from build123d import *

# Parameters (mm, degrees)
SKETCH001_W   = 60
SKETCH001_H   = 80
SKETCH001_W_2 = 56
SKETCH001_H_2 = 76
PAD_DEPTH     = 30


with BuildPart() as part:
    # Sketch001 → Pad (new body)
    with BuildSketch(Plane.XY.offset(2)):
        Rectangle(SKETCH001_W, SKETCH001_H)
        Rectangle(SKETCH001_W_2, SKETCH001_H_2, mode=Mode.SUBTRACT)
    extrude(amount=PAD_DEPTH)


solid = part.part
The listing builds one solid part. Answer for the finished solid, in the listing's coordinates (mm). A direction names the side the tool comes from. Coordinates: 2 decimals unless noted, no trailing zeros. Loops run counter-clockwise (first coordinate to the right, second up) from the corner with the lowest first, then second, coordinate; pieces in that order, holes last. Notation, with made-up numbers: (50.25, -39) -> (100.25, -39) arc R14 ccw to (100.25, -13) -> close; hole circle Ø3 at (12.5, 72). An arc over 180 degrees is marked (long way). Write item = value, one per line. Start each with the question number.
1) Straight lines are drawn through the part: line 1 (Y direction, x = -4, z = 15.5); line 2 (X direction, y = 20.5, z = 12.75). For each, find the intervals that lie inside material, in ascending order. Write a range as from..to.
2) A cutting plane is placed at A-A (z = 23.5). Give the vertices of the cut face in (x, y).
3) A tool of negligible diameter and unlimited length cuts with its end or side. For faces 1 (the face through (28, -1, 17)), 2 (the face through (-29, 0, 2)), from which of +Z, -Z, +X, -X, +Y, -Y can it reach the whole face along a straight path? Write none if from no direction.
4) A cutting plane is placed at B-B (x = -14.5). Give the vertices of the cut face in (y, z).
5) The mould has two halves that part along X. Classify faces 3 (the face through (-30, -1, 17)), 4 (the face through (0, -40, 17)), 5 (the face through (-28, -1, 17)): released by +X, released by -X, zero draft, split by the parting line, or undercut.
6) A cutting plane is placed at C-C (y = -34.5). Give the vertices of the cut face in (x, z), then the cut area to 3 significant figures.
Responses:
q1.line_1 = -40..-38, 38..40
q1.line_2 = -30..-28, 28..30
q2.outline = (-30, -40) -> (30, -40) -> (30, 40) -> (-30, 40) -> close; hole (-28, -38) -> (28, -38) -> (28, 38) -> (-28, 38) -> close
q3.face_1 = +Z, -Z
q3.face_2 = -Z, +X, -X, +Y, -Y
q4.outline = (-40, 2) -> (-38, 2) -> (-38, 32) -> (-40, 32) -> close; (38, 2) -> (40, 2) -> (40, 32) -> (38, 32) -> close
q5.face_3 = released by -X
q5.face_4 = zero draft
q5.face_5 = undercut
q6.outline = (-30, 2) -> (-28, 2) -> (-28, 32) -> (-30, 32) -> close; (28, 2) -> (30, 2) -> (30, 32) -> (28, 32) -> close
q6.area = 120 mm²
